Could you check a few things on this model? Use its own coordinates, in mm. A direction names the side the tool comes from. Give positions to 0.01 mm unless a question says otherwise; leave off trailing zeros. Order: outer loops, then holes, each group sorted by start corner. A loop starts at its lowest first (then second) coordinate and runs counter-clockwise, first axis right, second up. Notation, with made-up numbers: (-2, 26.25) - (56, 26.25) arc R20 cw to (56, 37.25) - close; hole circle Ø11 at (-21, -29). An arc over 180 degrees is marked (long way). One line per question, with ' | ' between items. Start each with the question number.
1. Imagine slicing it at A-A (y = 0). Please give me the cut outline in (x, z).
2. Imagine slicing it at C-C (x = -21). Please give me the cut outline in (y, z) (3 decimals), and give its area (3 significant figures).
3. I need wall thicknesses on probe 1 along X at (y, z) = (15, -7); probe 2 along X at (y, z) = (-7, -4); probe 3 along Z at (x, y) = (17.5, 9). Which ranges of each line are inside material? Lowest first, please. Write a range as from..to.
4. If we mould it in two halves opening along Y, with no side actions, what happens to faces 1 (the flat face through (25, -5, -11)), 2 (the flat face through (22, 10, 12)), 3 (the flat face through (7, -8, 6)), 4 (the flat face through (5, 0, 5))? For each: released by +Y, released by -Y, zero draft, split by the parting line, or undercut.
5. Imagine slicing it at B-B (z = -12). Please give me the cut outline in (x, y).
6. Which directions (+Z, -Z, +X, -X, +Y, -Y) give clear straight access to the entire face, cutting with the end or side of a thin tool? Please do faces 5 (the flat face through (10, -11, -2)), 6 (the flat face through (7, -10, 12)), 7 (the flat face through (0, 0, 18)), 8 (the flat face through (-50, 0, 5)), 9 (the flat face through (40, 9, -6)).
7. Imagine slicing it at D-D (y = -4). Please give me the cut outline in (x, z).
8. For P1, Ø6, axis at x = 29.5, z = 4.5, coming from the -Y side; P2, Ø4, axis at x = 8.5, y = -9.5, coming from the +Z side; P3, Ø5, axis at x = 20.5, z = -13, coming from the -Y side, each with a flat end and sliding along its axis, tell me the tip position at first contact or that it passes through.
```python
from build123d import *

# Parameters (mm, degrees)
F1_DEPTH = 5
F3_DEPTH = 35
F5_DEPTH = 5
F6_DEPTH = 10
F7_DEPTH = 50


with BuildPart() as f1:
    # F0 (on Right) → F1 (new body)
    with BuildSketch(Plane.YZ):
        with BuildLine():
            ThreePointArc((17.5, 0), (16.5770023354, 5.6082968512), (13.9053721633, 10.625))
            ThreePointArc((13.9053721633, 10.625), (14.7238001625, 7.8652589369), (15, 5))
            ThreePointArc((15, 5), (8.6602540378, -7.2474487139), (-5, -9.1421356237))
            Line((-5, -9.1421356237), (-5, -16.7705098312))
            ThreePointArc((-5, -16.7705098312), (10.4582503317, -14.0312152004), (17.5, 0))
        make_face()
        with BuildLine():
            ThreePointArc((13.9053721633, 10.625), (13.3392841662, 11.3275548082), (12.7377392029, 12))
            Line((12.7377392029, 12), (8, 12))
            Line((8, 12), (8, 0))
            ThreePointArc((8, 0), (3.4641016151, -7.2111025509), (-5, -6.2449979984))
            Line((-5, -6.2449979984), (-5, -9.1421356237))
            ThreePointArc((-5, -9.1421356237), (8.6602540378, -7.2474487139), (15, 5))
            ThreePointArc((15, 5), (14.7238001625, 7.8652589369), (13.9053721633, 10.625))
        make_face()
        with BuildLine():
            Line((8, 12), (12.7377392029, 12))
            ThreePointArc((12.7377392029, 12), (0, 17.5), (-12.7377392029, 12))
            Line((-12.7377392029, 12), (-8, 12))
            Line((-8, 12), (-8, 0))
            ThreePointArc((-8, 0), (-7.2111025509, -3.4641016151), (-5, -6.2449979984))
            ThreePointArc((-5, -6.2449979984), (3.4641016151, -7.2111025509), (8, 0))
            Line((8, 0), (8, 12))
        make_face()
        with BuildLine():
            Line((-8, 12), (-12.7377392029, 12))
            ThreePointArc((-12.7377392029, 12), (-13.3392841662, 11.3275548082), (-13.9053721633, 10.625))
            ThreePointArc((-13.9053721633, 10.625), (-13.6761905094, -1.1613158619), (-5, -9.1421356237))
            Line((-5, -9.1421356237), (-5, -6.2449979984))
            ThreePointArc((-5, -6.2449979984), (-7.2111025509, -3.4641016151), (-8, 0))
            Line((-8, 0), (-8, 12))
        make_face()
        with BuildLine():
            ThreePointArc((-5, -9.1421356237), (-13.6761905094, -1.1613158619), (-13.9053721633, 10.625))
            ThreePointArc((-13.9053721633, 10.625), (-16.6427691172, -5.4100125798), (-5, -16.7705098312))
            Line((-5, -16.7705098312), (-5, -9.1421356237))
        make_face()
    extrude(amount=F1_DEPTH)

    # F2 (on face) → F3 (join)
    with BuildSketch(Plane.YZ.offset(5)):
        with BuildLine():
            ThreePointArc((15, 5), (8.6602540378, -7.2474487139), (-5, -9.1421356237))
            Line((-5, -9.1421356237), (-5, -16.7705098312))
            ThreePointArc((-5, -16.7705098312), (10.4582503317, -14.0312152004), (17.5, 0))
            ThreePointArc((17.5, 0), (16.5770023354, 5.6082968512), (13.9053721633, 10.625))
            ThreePointArc((13.9053721633, 10.625), (14.7238001625, 7.8652589369), (15, 5))
        make_face()
        with BuildLine():
            ThreePointArc((8, 0), (3.4641016151, -7.2111025509), (-5, -6.2449979984))
            Line((-5, -6.2449979984), (-5, -9.1421356237))
            ThreePointArc((-5, -9.1421356237), (8.6602540378, -7.2474487139), (15, 5))
            ThreePointArc((15, 5), (14.7238001625, 7.8652589369), (13.9053721633, 10.625))
            ThreePointArc((13.9053721633, 10.625), (13.3392841662, 11.3275548082), (12.7377392029, 12))
            Line((12.7377392029, 12), (8, 12))
            Line((8, 12), (8, 0))
        make_face()
    extrude(amount=F3_DEPTH)

    # F4 (on face) → F5 (join)
    with BuildSketch(Plane.YZ.offset(5)):
        with BuildLine():
            ThreePointArc((-13.9053721633, 10.625), (-16.6427691172, -5.4100125798), (-5, -16.7705098312))
            Line((-5, -16.7705098312), (-5, -9.1421356237))
            ThreePointArc((-5, -9.1421356237), (-13.6761905094, -1.1613158619), (-13.9053721633, 10.625))
        make_face()
        with BuildLine():
            ThreePointArc((-13.9053721633, 10.625), (-13.6761905094, -1.1613158619), (-5, -9.1421356237))
            Line((-5, -9.1421356237), (-5, -6.2449979984))
            ThreePointArc((-5, -6.2449979984), (-7.2111025509, -3.4641016151), (-8, 0))
            Line((-8, 0), (-8, 12))
            Line((-8, 12), (-12.7377392029, 12))
            ThreePointArc((-12.7377392029, 12), (-13.3392841662, 11.3275548082), (-13.9053721633, 10.625))
        make_face()
    extrude(amount=F5_DEPTH)

    # F0 (on Right) → F6 (join)
    with BuildSketch(Plane.YZ):
        with BuildLine():
            ThreePointArc((-5, -9.1421356237), (-13.6761905094, -1.1613158619), (-13.9053721633, 10.625))
            ThreePointArc((-13.9053721633, 10.625), (-16.6427691172, -5.4100125798), (-5, -16.7705098312))
            Line((-5, -16.7705098312), (-5, -9.1421356237))
        make_face()
    extrude(amount=-F6_DEPTH)

    # F0 (on Right) → F7 (join)
    with BuildSketch(Plane.YZ):
        with BuildLine():
            ThreePointArc((-12.7377392029, 12), (0, 17.5), (12.7377392029, 12))
            ThreePointArc((12.7377392029, 12), (13.3392841662, 11.3275548082), (13.9053721633, 10.625))
            ThreePointArc((13.9053721633, 10.625), (0, 20), (-13.9053721633, 10.625))
            ThreePointArc((-13.9053721633, 10.625), (-13.3392841662, 11.3275548082), (-12.7377392029, 12))
        make_face()
        with BuildLine():
            Line((8, 12), (12.7377392029, 12))
            ThreePointArc((12.7377392029, 12), (0, 17.5), (-12.7377392029, 12))
            Line((-12.7377392029, 12), (-8, 12))
            Line((-8, 12), (-8, 0))
            ThreePointArc((-8, 0), (-7.2111025509, -3.4641016151), (-5, -6.2449979984))
            ThreePointArc((-5, -6.2449979984), (3.4641016151, -7.2111025509), (8, 0))
            Line((8, 0), (8, 12))
        make_face()
        with BuildLine():
            Line((-8, 12), (-12.7377392029, 12))
            ThreePointArc((-12.7377392029, 12), (-13.3392841662, 11.3275548082), (-13.9053721633, 10.625))
            ThreePointArc((-13.9053721633, 10.625), (-13.6761905094, -1.1613158619), (-5, -9.1421356237))
            Line((-5, -9.1421356237), (-5, -6.2449979984))
            ThreePointArc((-5, -6.2449979984), (-7.2111025509, -3.4641016151), (-8, 0))
            Line((-8, 0), (-8, 12))
        make_face()
        with BuildLine():
            ThreePointArc((13.9053721633, 10.625), (13.3392841662, 11.3275548082), (12.7377392029, 12))
            Line((12.7377392029, 12), (8, 12))
            Line((8, 12), (8, 0))
            ThreePointArc((8, 0), (3.4641016151, -7.2111025509), (-5, -6.2449979984))
            Line((-5, -6.2449979984), (-5, -9.1421356237))
            ThreePointArc((-5, -9.1421356237), (8.6602540378, -7.2474487139), (15, 5))
            ThreePointArc((15, 5), (14.7238001625, 7.8652589369), (13.9053721633, 10.625))
        make_face()
    extrude(amount=-F7_DEPTH)


solid = f1.part
```
Results found:
1) outline: (-50, -10) - (0, -10) - (0, -17.5) - (40, -17.5) - (40, -8) - (5, -8) - (5, 17.5) - (0, 17.5) - (0, 20) - (-50, 20) - close
2) outline: circle Ø30 at (0, 5) | area: 707 mm2
3) probe 1: x = 0..40 | probe 2: x = -50..10 | probe 3: z = -15.01..12
4) face 1: released by -Y | face 2: zero draft | face 3: undercut | face 4: undercut
5) outline: (-10, -12.74) - (10, -12.74) - (10, -5) - (40, -5) - (40, 12.74) - (0, 12.74) - (0, -5) - (-10, -5) - close
6) face 5: +Z, -Z, +X, -Y | face 6: +Z, +X, +Y, -Y | face 7: +Z, +X | face 8: +Z, -Z, -X, +Y, -Y | face 9: +Z, -Z, +X, +Y, -Y
7) outline: (-50, -9.46) - (0, -9.46) - (0, -17.04) - (40, -17.04) - (40, -6.93) - (5, -6.93) - (5, 17.04) - (0, 17.04) - (0, 19.46) - (-50, 19.46) - close
8) P1: stops at y = 8 | P2: stops at z = 12 | P3: stops at y = -5
